Job drawing, mm, ordinate dimensions from the low corner. One solid piece. A direction names the side the tool comes from. Round coordinates to 2 decimals unless told otherwise and drop trailing zeros. Order: outer loops, then holes, each group sorted by start corner. A loop starts at its lowest first (then second) coordinate and runs counter-clockwise, first axis right, second up. Notation, with made-up numbers: (41, 85) -> (52, 85) arc R22 ccw to (52, 100) -> close; hole circle Ø10 at (52, 9.25). An arc over 180 degrees is marked (long way). Return JSON: item names as keys, results as strings. Group by question number.
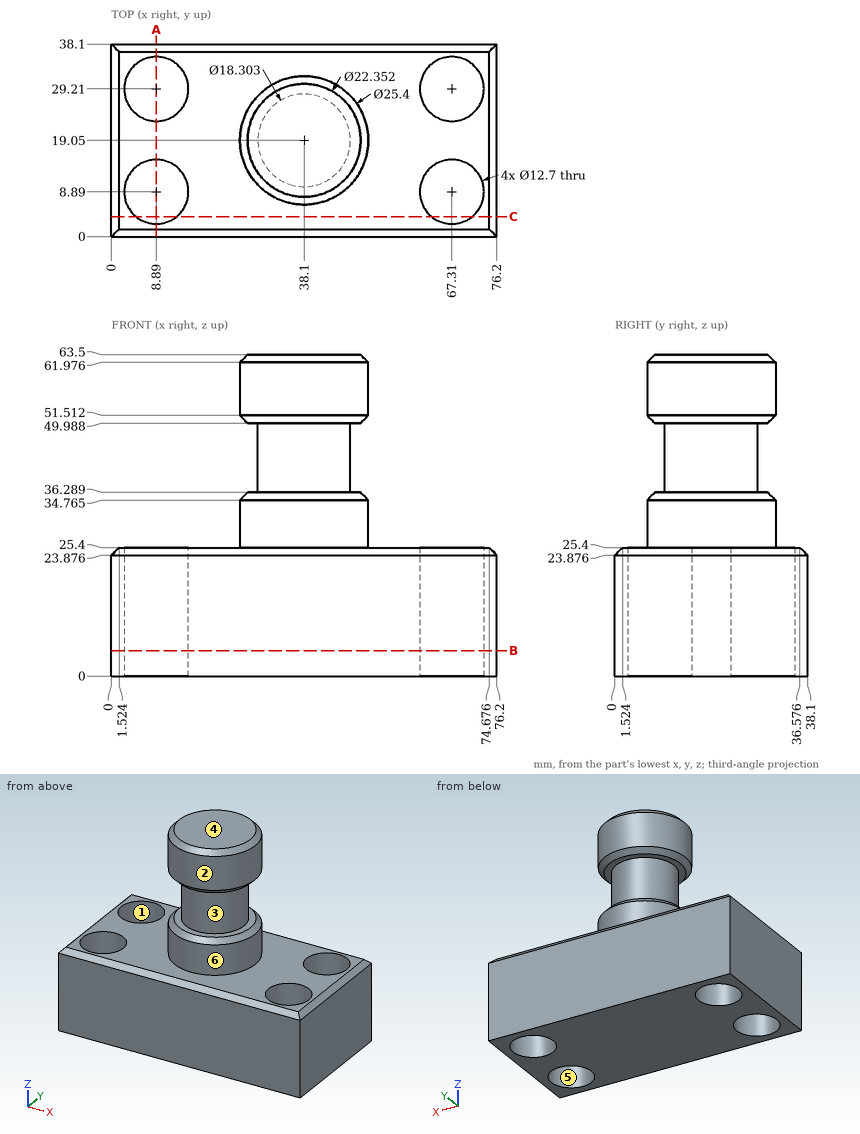
(1) Saw through at A-A, the plane x = 8.89. List the corners of the cut face in (y, z).
(2) Probe L1, parallel to Y at x = 67.31, z = 15.75; L2, parallel to X at y = 29, z = 18; L3, parallel to Y at x = 8, z = 19. List the from-to ranges inside material, lowest first. Write a range as [from, to].
(3) Tool access for the marked faces 1, 2 and 3: list every direction of +Z, -Z, +X, -X, +Y, -Y with a clear straight run to the whole face (end or side of a thin tool).
(4) Pin check, flat tips, straight feed: P1, Ø2, axis at y = 28.5, z = 34, coming from the -X side; P2, Ø10, axis at x = 8.89, y = 8.89, coming from the -Z side; P3, Ø16.5, axis at x = 8.89, y = 29.21, coming from the +Z side; P4, Ø2, axis at x = 38, z = 37.5, coming from the +Y side. Stop position of each tip, or through.
(5) Saw through at B-B, the plane z = 5. List the corners of the cut face in (x, y), and give its area (3 significant figures).
(6) Mould opens along Y. For the marked faces 4, 5 and 6 say: pulls with the +Y half, pulls with the -Y half, needs draft (parallel to the pull), parting line crosses it, or undercut.
(7) Saw through at C-C, the plane y = 4. List the corners of the cut face in (x, z), and give its area (3 significant figures).
Results are:
{
 "1": {"outline": "(0, 0) -> (2.54, 0) -> (2.54, 25.4) -> (1.52, 25.4) -> (0, 23.88) -> close; (15.24, 0) -> (22.86, 0) -> (22.86, 25.4) -> (15.24, 25.4) -> close; (35.56, 0) -> (38.1, 0) -> (38.1, 23.88) -> (36.58, 25.4) -> (35.56, 25.4) -> close"},
 "2": {"L1": "y = [0, 2.54], [15.24, 22.86], [35.56, 38.1]", "L2": "x = [0, 2.54], [15.24, 60.96], [73.66, 76.2]", "L3": "y = [0, 2.6], [15.18, 22.92], [35.5, 38.1]"},
 "3": {"face 1": "+Z, -Z", "face 2": "+Z", "face 3": "none"},
 "4": {"P1": "stops at x = 28.62", "P2": "passes through", "P3": "stops at z = 25.4", "P4": "stops at y = 28.2"},
 "5": {"outline": "(0, 0) -> (76.2, 0) -> (76.2, 38.1) -> (0, 38.1) -> close; hole circle Ø12.7 at (8.89, 8.89); hole circle Ø12.7 at (8.89, 29.21); hole circle Ø12.7 at (67.31, 8.89); hole circle Ø12.7 at (67.31, 29.21)", "area": "2,400 mm^2"},
 "6": {"face 4": "needs draft", "face 5": "undercut", "face 6": "parting line crosses it"},
 "7": {"outline": "(0, 0) -> (4.84, 0) -> (4.84, 25.4) -> (1.52, 25.4) -> (0, 23.88) -> close; (12.94, 0) -> (63.26, 0) -> (63.26, 25.4) -> (12.94, 25.4) -> close; (71.36, 0) -> (76.2, 0) -> (76.2, 23.88) -> (74.68, 25.4) -> (71.36, 25.4) -> close", "area": "1,520 mm^2"}
}
